Autodesk Inventor part; units mm, degrees
ref_plane "YZ Plane" through (0, 0, 0) normal (1, 0, 0) x (0, 1, 0)
ref_plane "XZ Plane" through (0, 0, 0) normal (0, 1, 0) x (-1, 0, 0)
ref_plane "XY Plane" through (0, 0, 0) normal (0, 0, 1) x (1, 0, 0)
sketch "Sketch1" plane through (0, 0, 0) normal (0, 1, 0) x (-1, 0, 0)
  line L0 (0, 0) -> (95, 0)
  line L1 (95, 0) -> (95, -95)
  line L2 (95, -95) -> (0, -95)
  line L3 (0, -95) -> (0, 0)
  dimension "d0" = 95
  dimension "d1" = 95
extrude "Extrusion1" add sketch "Sketch1" along normal blind 5
chamfer "Chamfer1" distance 10 angle 45 4 edges at (0, 2.5, -95) (0, 2.5, 0) (-95, 2.5, 0) (-95, 2.5, -95)
sketch "Sketch2" plane through (0, 0, 0) normal (0, -1, 0) x (1, 0, 0)
  line L0 (-85, -95) -> (-95, -85)
  line L1 (-10, -95) -> (-85, -95)
  line L2 (0, -85) -> (-10, -95)
  line L3 (0, -10) -> (0, -85)
  line L4 (-10, 0) -> (0, -10)
  line L5 (-85, 0) -> (-10, 0)
  line L6 (-95, -10) -> (-85, 0)
  line L7 (-95, -85) -> (-95, -10)
  line L8 (-47.5, -95) -> (-47.5, -71.232)
  line L9 (-47.5, -71.232) -> (-35, -71.232)
  circle A0 centre (-35, -71.232) radius 2.5
  circle A1 centre (-60, -71.232) radius 2.5
  point P0 (0, 0)
  dimension "d7" = 23.768
  dimension "d9" = 12.5
  dimension "d15" = 5
extrude "Extrusion2" cut sketch "Sketch2" against normal blind 5 contours A0 | A1
sketch "Sketch3" plane through (0, 0, 0) normal (0, -1, 0) x (1, 0, 0)
  circle A0 centre (-35, -71.232) radius 2.5
  line L0 (-85, -95) -> (-95, -85)
  line L1 (-10, -95) -> (-85, -95)
  line L2 (0, -85) -> (-10, -95)
  line L3 (0, -10) -> (0, -85)
  line L4 (-10, 0) -> (0, -10)
  line L5 (-85, 0) -> (-10, 0)
  line L6 (-95, -10) -> (-85, 0)
  line L7 (-95, -85) -> (-95, -10)
  line L8 (-47.5, -95) -> (-47.5, -47.5)
  line L9 (-85, 0) -> (-10, 0)
  line L10 (-34.5, -47.5) -> (-60.5, -47.5)
  circle A1 centre (-34.5, -47.5) radius 8
  circle A2 centre (-60.5, -47.5) radius 8
  point P0 (0, 0)
  dimension "d17" = 47.5
  dimension "d18" = 26
  dimension "d19" = 16
extrude "Extrusion3" cut sketch "Sketch3" against normal blind 5 contours A1 | A2
sketch "Sketch4" plane through (0, 0, 0) normal (0, -1, 0) x (1, 0, 0)
  circle A0 centre (-60.5, -47.5) radius 8
  circle A1 centre (-34.5, -47.5) radius 8
  circle A2 centre (-35, -71.232) radius 2.5
  line L0 (-85, -95) -> (-95, -85)
  line L1 (-10, -95) -> (-85, -95)
  line L2 (0, -85) -> (-10, -95)
  line L3 (0, -10) -> (0, -85)
  line L4 (-10, 0) -> (0, -10)
  line L5 (-85, 0) -> (-10, 0)
  line L6 (-95, -10) -> (-85, 0)
  line L7 (-95, -85) -> (-95, -10)
  line L8 (-47.5, -95) -> (-47.5, -47.5)
  line L9 (-85, 0) -> (-10, 0)
  line L10 (-70, -57.5) -> (-25, -57.5)
  line L11 (-25, -57.5) -> (-25, -37.5)
  line L12 (-25, -37.5) -> (-70, -37.5)
  line L13 (-70, -37.5) -> (-70, -57.5)
  line L14 (-70, -57.5) -> (-25, -37.5) construction
  line L15 (-25, -57.5) -> (-70, -37.5) construction
  line L16 (-22, -34.5) -> (-22, -60.5)
  line L17 (-22, -60.5) -> (-73, -60.5)
  line L18 (-73, -60.5) -> (-73, -34.5)
  line L19 (-73, -34.5) -> (-22, -34.5)
  line L20 (-25, -57.5) -> (-25, -60.5)
  line L21 (-70, -57.5) -> (-70, -60.5)
  point P0 (0, 0)
  point P1 (-70, -60.5)
  dimension "d22" = 47.5
  dimension "d23" = 45
  dimension "d24" = 20
  dimension "d25" = 3
extrude "Extrusion4" add sketch "Sketch4" along normal blind 11.2 contours L20 L11 L12 L13 L21 L17 L18 L19 L16
sketch "Sketch5" plane through (0, -11.2, 0) normal (0, -1, 0) x (1, 0, 0)
  line L0 (-70, -37.5) -> (-25, -37.5)
  line L1 (-25, -37.5) -> (-25, -60.5)
  line L2 (-25, -60.5) -> (-22, -60.5)
  line L3 (-22, -60.5) -> (-22, -34.5)
  line L4 (-22, -34.5) -> (-73, -34.5)
  line L5 (-73, -34.5) -> (-73, -60.5)
  line L6 (-73, -60.5) -> (-70, -60.5)
  line L7 (-70, -60.5) -> (-70, -37.5)
  line L8 (-25, -60.5) -> (-70, -60.5)
  point P0 (0, 0)
extrude "Extrusion5" add sketch "Sketch5" against normal blind 3 contours L0 L1 L8 L7
sketch "Sketch6" plane through (0, -11.2, 0) normal (0, -1, 0) x (1, 0, 0)
  line L0 (-25, -37.5) -> (-70, -37.5)
  line L1 (-70, -37.5) -> (-70, -60.5)
  line L2 (-25, -60.5) -> (-25, -37.5)
  line L3 (-70, -37.5) -> (-70, -39.25)
  line L4 (-70, -39.25) -> (-68, -39.25)
  circle A0 centre (-68, -39.25) radius 1.5
  line L5 (-47.5, -37.5) -> (-47.5, -39.5)
  circle A1 centre (-27, -39.25) radius 1.5
  line L6 (-73, -60.5) -> (-22, -60.5)
  line L7 (-47.5, -60.5) -> (-57.5, -60.5)
  line L8 (-57.5, -60.5) -> (-57.5, -52.5)
  line L9 (-57.5, -52.5) -> (-47.5, -52.5)
  line L10 (-47.5, -52.5) -> (-47.5, -60.5)
  line L11 (-37.5, -60.5) -> (-37.5, -52.5)
  line L12 (-37.5, -52.5) -> (-47.5, -52.5)
  point P0 (0, 0)
  dimension "d30" = 1.75
  dimension "d31" = 2
  dimension "d32" = 3
  dimension "d33" = 2
  dimension "d36" = 10
  dimension "d37" = 8
extrude "Extrusion6" cut sketch "Sketch6" against normal blind 3 contours L6 L10 L12 L11 | L6 L8 L9 L10 | A0 | A1
fillet "Fillet1" radius 2 16 edges at (-90, 0, -5) (-95, 0, -47.5) (-47.5, 0, 0) (-5, 0, -5) (0, 0, -47.5) (-90, 0, -90) (-47.5, 0, -95) (-5, 0, -90) (-22, -11.2, -47.5) (-47.5, -11.2, -34.5) (-73, -11.2, -47.5) (-65.25, -11.2, -60.5) (-29.75, -11.2, -60.5) (-47.5, -11.2, -52.5) (-57.5, -11.2, -56.5) (-37.5, -11.2, -56.5)
properties part number "TutupAtas"
For this review, take the finished solid that the model builds, in its own axes (mm). A direction names the side the tool comes from. Round coordinates to 2 decimals unless told otherwise and drop trailing zeros. Order: outer loops, then holes, each group sorted by start corner. A loop starts at its lowest first (then second) coordinate and runs counter-clockwise, first axis right, second up. Notation, with made-up numbers: (41, 81.5) -> (95, 81.5) arc R35 cw to (95, 117.5) -> close; hole circle Ø6 at (1.25, 47.5). An arc over 180 degrees is marked (long way). Use a Markdown table: item, result.
Item 1: Take a section at C-C (y = -6.25). State the section outline as (x, z) points.
Resolved:
| item | result |
|---|---|
| outline | (-73, -60.5) -> (-70, -60.5) -> (-70, -37.5) -> (-25, -37.5) -> (-25, -60.5) -> (-22, -60.5) -> (-22, -34.5) -> (-73, -34.5) -> close |
Item 2: For pin 1 (3 mm diameter, centred on x = -31, y = -3.5, fed in from -Z); pin 2 (1 mm diameter, centred on y = 0, z = -34, fed in from +X); pin 3 (2.5 mm diameter, centred on y = -4, z = -43.5, fed in from +X), all flat-tipped, find the tip position at first contact; note any pin that passes through.
Resolved:
| item | result |
|---|---|
| pin 1 | stops at z = -37.5 |
| pin 2 | stops at x = -0.68 |
| pin 3 | stops at x = -22 |
Item 3: Take a section at A-A (x = -48.5). State the section outline as (y, z) points.
Resolved:
| item | result |
|---|---|
| outline | (-11.2, -50.5) arc R2 ccw to (-9.2, -52.5) -> (-8.2, -52.5) -> (-8.2, -37.5) -> (0, -37.5) -> (0, -93) arc R2 ccw to (2, -95) -> (5, -95) -> (5, 0) -> (2, 0) arc R2 ccw to (0, -2) -> (0, -34.5) -> (-9.2, -34.5) arc R2 ccw to (-11.2, -36.5) -> close |
Item 4: Draft analysis for pull direction X (two halves, no side actions). For faces 1 (the flat face through (-5, 4, -5)), 2 (the cylindrical face through (-61.541, 2.465, -39.568)), 3 (the flat face through (-24.5, -6, -60.5)), state which applies: +X half, -X half, draft (parallel to the pull), parting line (faces both ways), or undercut.
Resolved:
| item | result |
|---|---|
| face 1 | +X half |
| face 2 | undercut |
| face 3 | draft |
Item 5: Take a section at B-B (z = -81). State the section outline as (x, y) points, plus the area to 3 significant figures.
Resolved:
| item | result |
|---|---|
| outline | (-95, 2) arc R2 ccw to (-93, 0) -> (-2, 0) arc R2 ccw to (0, 2) -> (0, 5) -> (-95, 5) -> close |
| area | 473 mm² |
Item 6: Take a section at D-D (x = -64). State the section outline as (y, z) points, plus the area to 3 significant figures.
Resolved:
| item | result |
|---|---|
| outline | (-11.2, -58.5) arc R2 ccw to (-9.2, -60.5) -> (-8.2, -60.5) -> (-8.2, -37.5) -> (0, -37.5) -> (0, -40.31) -> (5, -40.31) -> (5, 0) -> (2, 0) arc R2 ccw to (0, -2) -> (0, -34.5) -> (-9.2, -34.5) arc R2 ccw to (-11.2, -36.5) -> close; (0, -93) arc R2 ccw to (2, -95) -> (5, -95) -> (5, -54.69) -> (0, -54.69) -> close |
| area | 502 mm² |
Item 7: Machinability: for faces 4 (the flat face through (-47, -4, -37.5)), 5 (the cylindrical face through (-28.19, -9.72, -40.16)), 6 (the flat face through (-73, -5, -48)), which of the approach directions +Z, -Z, +X, -X, +Y, -Y give a long, thin tool a straight path to every point of the face, cutting with its end or side? Answer none if there is none.
Resolved:
| item | result |
|---|---|
| face 4 | -Z |
| face 5 | -Y |
| face 6 | +Z, -Z, -X, -Y |
Item 8: For line 1 along Z through (x, y) = (-60, 3.55); line 2 along Z through (x, y) = (-60.5, 2.9); line 3 along X through (y, z) = (-6.75, -45), list the stretches that pass through material, from the lowest coordinate up. Write a range as [from, to].
Resolved:
| item | result |
|---|---|
| line 1 | z = [-95, -73.73], [-68.73, -55.48], [-39.52, 0] |
| line 2 | z = [-95, -73.68], [-68.78, -55.5], [-39.5, 0] |
| line 3 | x = [-73, -70], [-25, -22] |
